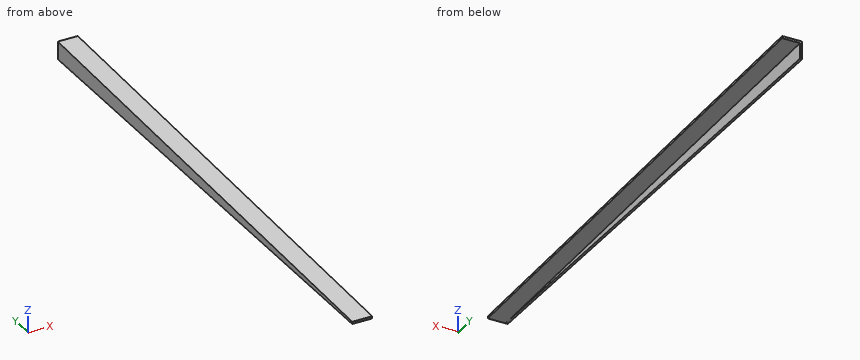
from build123d import *

# Parameters (mm, degrees)
F1_DEPTH = 6.35
F3_DEPTH = 50.8


with BuildPart() as f1:
    # F0 (on Right) → F1 (new body)
    with BuildSketch(Plane.YZ):
        Polygon((-748.298248, -6.35), (763.001752, -6.35), (763.001752, 44.45), (-748.298248, 0), align=None)
    extrude(amount=F1_DEPTH)

    # F2 (on face) → F3 (join)
    with BuildSketch(Plane.YZ.offset(6.35)):
        Polygon((-748.298248, -6.35), (763.001752, 38.1), (763.001752, 44.45), (-748.298248, 0), align=None)
    extrude(amount=F3_DEPTH)


solid = f1.part
Check sheet for the modelled part. Datum: model origin and axes. Units: mm. Round coordinates to 2 decimals unless told otherwise and drop trailing zeros. Order: outer loops, then holes, each group sorted by start corner. A loop starts at its lowest first (then second) coordinate and runs counter-clockwise, first axis right, second up. Notation, with made-up numbers: M 28,30 L 39,30 A28 cw 39,48 Z; hole C -7,7 d10. An arc over 180 degrees is marked long. One line per item, written item: value. Start each with the question number.
1. Section check C-C on x = 25. Enter the section's corners in (y, z).
2. Scan lines: line 1 along X through (y, z) = (640, 10); line 2 along Z through (x, y) = (25.5, 435); line 3 along Z through (x, y) = (30, -541). Record each from-to range of solid material in increasing order.
3. Section check A-A on z = 23. Enter the section's corners in (x, y), and give its area (3 significant figures).
4. Section check B-B on y = 517.5. Enter the section's corners in (x, z).
5. Gauge pin test, flat ends, axial feed: P1, Ø8, axis at x = 20, y = 311.5, coming from the +Z side; P2, Ø8, axis at x = 23.5, y = -478.5, coming from the +Z side; P3, Ø6, axis at x = 12.5, y = -206, coming from the +Z side. Record the tip position at first contact, or that the pin passes through.
Results found:
1. outline: M -748.3,-6.35 L 763,38.1 L 763,44.45 L -748.3,0 Z
2. line 1: 0 to 6.35
2. line 2: 28.45 to 34.8
2. line 3: -0.25 to 6.1
3. outline: M 0,33.7 L 57.15,33.7 L 57.15,249.6 L 6.35,249.6 L 6.35,763 L 0,763 Z
3. area: 15,600 mm^2
4. outline: M 0,-6.35 L 6.35,-6.35 L 6.35,30.88 L 57.15,30.88 L 57.15,37.23 L 0,37.23 Z
5. P1: z = 31.29
5. P2: z = 8.05
5. P3: z = 16.04
